Source: CAD feature listing. Evaluate the final solid. Frame: model axes, mm. Give positions to 0.01 mm unless a question says otherwise; leave off trailing zeros. Order: outer loops, then holes, each group sorted by start corner. A loop starts at its lowest first (then second) coordinate and runs counter-clockwise, first axis right, second up. Notation, with made-up numbers: (20, 42) - (33, 42) arc R22 ccw to (33, 51) - close; hole circle Ø4 at (-22, 59). An arc over 180 degrees is marked (long way). One line per item, written item: value. Start each with the question number.
Autodesk Inventor part; units mm, degrees
ref_plane "YZ Plane" through (0, 0, 0) normal (1, 0, 0) x (0, 1, 0)
ref_plane "XZ Plane" through (0, 0, 0) normal (0, 1, 0) x (-1, 0, 0)
ref_plane "XY Plane" through (0, 0, 0) normal (0, 0, 1) x (1, 0, 0)
sketch "Sketch1" plane through (0, 0, 0) normal (0, 0, 1) x (1, 0, 0)
  circle A0 centre (0, 0) radius 6.475
  arc A1 (-12.5, 0) -> (12.5, 0) centre (0, 0) ccw
  line L0 (-12.5, 0) -> (-12.5, 22)
  line L1 (-12.5, 22) -> (12.5, 22)
  line L2 (12.5, 22) -> (12.5, 0)
  dimension "d0" = 12.95
  dimension "d1" = 25
  dimension "d2" = 22
  dimension "d3" = 25
extrude "Extrusion1" add sketch "Sketch1" along normal blind 6
sketch "Sketch3" plane through (0, 0, 6) normal (0, 0, 1) x (1, 0, 0)
  circle A0 centre (-8, 0) radius 0.75
  circle A1 centre (8, 0) radius 0.75
  point P0 (0, 0)
  dimension "d7" = 16
  dimension "d8" = 8
  dimension "d9" = 1.5
  dimension "d10" = 1.5
extrude "Extrusion2" cut sketch "Sketch3" against normal blind 8
properties part number "Bearing Housing"
1. Draft query along X for faces 1 (the flat face through (0, 9, 0)), 2 (the cylindrical face through (0.275, -12.497, 2.958)), 3 (the cylindrical face through (7.25, 0.03, 3.04)). Return one class per face: pulls with the +X half, pulls with the -X half, needs draft (parallel to the pull), parting line crosses it, or undercut.
2. Section B-B on z = 4.1. Return the cut outline in (x, y) (3 decimals), then the cut area to 3 significant figures.
3. Section C-C on y = 3.5. Return the cut outline in (x, z).
4. Section D-D on y = -9. Return the cut outline in (x, z), then the cut area to 3 significant figures.
5. Section A-A on x = 0. Return the cut outline in (y, z) (3 decimals).
6. Ray query, L1, parallel to Y at x = 0, z = 2.6 (3 decimals); L2, parallel to Y at x = 8, z = 4.5; L3, parallel to X at y = 5, z = 2. Return the intervals inside material, ascending.
7. Contact query for a flat-ended pin moving along its axis: pin 1 Ø4 at (x, y) = (4, 5) entering from +Z. Output: stop coordinate, or through.
Data:
1. face 1: needs draft
1. face 2: parting line crosses it
1. face 3: undercut
2. outline: (-12.5, 0) arc R12.5 ccw to (12.5, 0) - (12.5, 22) - (-12.5, 22) - close; hole circle Ø1.5 at (-8, 0); hole circle Ø12.95 at (0, 0); hole circle Ø1.5 at (8, 0)
2. area: 660 mm2
3. outline: (-12.5, 0) - (-5.45, 0) - (-5.45, 6) - (-12.5, 6) - close; (5.45, 0) - (12.5, 0) - (12.5, 6) - (5.45, 6) - close
4. outline: (-8.67, 0) - (8.67, 0) - (8.67, 6) - (-8.67, 6) - close
4. area: 104 mm2
5. outline: (-12.5, 0) - (-6.475, 0) - (-6.475, 6) - (-12.5, 6) - close; (6.475, 0) - (22, 0) - (22, 6) - (6.475, 6) - close
6. L1: y = -12.5 to -6.475, 6.475 to 22
6. L2: y = -9.6 to -0.75, 0.75 to 22
6. L3: x = -12.5 to -4.11, 4.11 to 12.5
7. pin 1: stops at z = 6
